from build123d import *

# Parameters (mm, degrees)
BOSS_EXTRUDE1_DEPTH     = 760
LPATTERN1_COUNT         = 2
LPATTERN1_PITCH         = 80
LPATTERN2_COUNT         = 9
LPATTERN2_PITCH         = 160
CUT_EXTRUDE1_DEPTH      = 40
CUT_EXTRUDE1_DEPTH_BACK = 20
SKETCH5_W               = 307.175258626
SKETCH5_H               = 1220.849909684


with BuildPart() as part:
    # Sketch1 → Boss-Extrude1 (new, symmetric)
    with BuildSketch(Plane.XY):
        with BuildLine():
            Line((-9.911771432, 13.106808119), (-11.43, 12.7))
            Line((-11.43, 12.7), (-14, 10.13))
            Line((-14, 10.13), (-14, 1.5))
            Line((-14, 1.5), (-12.5, 0))
            Line((-12.5, 0), (12.5, 0))
            Line((12.5, 0), (14, 1.5))
            Line((14, 1.5), (14, 10.13))
            Line((14, 10.13), (11.43, 12.7))
            Line((11.43, 12.7), (9.911771432, 13.106808119))
            ThreePointArc((9.911771432, 13.106808119), (9.10996999, 13.642554715), (8.8, 14.555696858))
            Line((8.8, 14.555696858), (8.8, 20.444303142))
            ThreePointArc((8.8, 20.444303142), (9.10996999, 21.357445285), (9.911771432, 21.893191881))
            Line((9.911771432, 21.893191881), (11.43, 22.3))
            Line((11.43, 22.3), (14, 24.87))
            Line((14, 24.87), (14, 26.5))
            ThreePointArc((14, 26.5), (13.416985894, 27.416985894), (12.5, 28))
            Line((12.5, 28), (-12.5, 28))
            ThreePointArc((-12.5, 28), (-13.416985894, 27.416985894), (-14, 26.5))
            Line((-14, 26.5), (-14, 24.87))
            Line((-14, 24.87), (-11.43, 22.3))
            Line((-11.43, 22.3), (-9.911771432, 21.893191881))
            ThreePointArc((-9.911771432, 21.893191881), (-9.10996999, 21.357445285), (-8.8, 20.444303142))
            Line((-8.8, 20.444303142), (-8.8, 14.555696858))
            ThreePointArc((-8.8, 14.555696858), (-9.10996999, 13.642554715), (-9.911771432, 13.106808119))
        make_face()
    extrude(amount=BOSS_EXTRUDE1_DEPTH, both=True)

    # Sketch2 → Cut-Revolve1 (revolve, cut)
    with BuildSketch(Plane(origin=(0, 0, 0), x_dir=(0, 0, -1), z_dir=(1, 0, 0)), mode=Mode.PRIVATE) as cut_revolve1_sk:
        Polygon((-720, 28), (-713, 28), (-713, 16), (-715.5, 16), (-715.5, 0), (-720, 0), align=None)
    cut_revolve1 = revolve(cut_revolve1_sk.sketch.rotate(Axis((0, 28, 720), (0, -1, 0)), 180), axis=Axis((0, 28, 720), (0, -1, 0)), mode=Mode.SUBTRACT)

    # LPattern1: Cut-Revolve1 ×2
    with Locations(*[(0, 0, -i * LPATTERN1_PITCH) for i in range(1, LPATTERN1_COUNT)]):
        add(cut_revolve1, mode=Mode.SUBTRACT)

    # Mirror1: Cut-Revolve1 across plane
    add(cut_revolve1.mirror(Plane.XY), mode=Mode.SUBTRACT)

    # Mirror1 copy 1 sketch → Mirror1 copy 1 (revolve, cut)
    with BuildSketch(Plane(origin=(0, 0, 80), x_dir=(0, 0, 1), z_dir=(1, 0, 0))):
        Polygon((-720, -28), (-713, -28), (-713, -16), (-715.5, -16), (-715.5, 0), (-720, 0), align=None)
    revolve(axis=Axis((0, 28, -640), (0, 1, 0)), mode=Mode.SUBTRACT)

    # LPattern2: Cut-Revolve1 ×9
    with Locations(*[(0, 0, -i * LPATTERN2_PITCH) for i in range(1, LPATTERN2_COUNT)]):
        add(cut_revolve1, mode=Mode.SUBTRACT)

    # LPattern2 copy 1 sketch → LPattern2 copy 1 (revolve, cut)
    with BuildSketch(Plane(origin=(0, 0, -240), x_dir=(0, 0, -1), z_dir=(1, 0, 0))):
        Polygon((-720, 28), (-713, 28), (-713, 16), (-715.5, 16), (-715.5, 0), (-720, 0), align=None)
    revolve(axis=Axis((0, 28, 480), (0, -1, 0)), mode=Mode.SUBTRACT)

    # LPattern2 copy 2 sketch → LPattern2 copy 2 (revolve, cut)
    with BuildSketch(Plane(origin=(0, 0, -400), x_dir=(0, 0, -1), z_dir=(1, 0, 0))):
        Polygon((-720, 28), (-713, 28), (-713, 16), (-715.5, 16), (-715.5, 0), (-720, 0), align=None)
    revolve(axis=Axis((0, 28, 320), (0, -1, 0)), mode=Mode.SUBTRACT)

    # LPattern2 copy 3 sketch → LPattern2 copy 3 (revolve, cut)
    with BuildSketch(Plane(origin=(0, 0, -560), x_dir=(0, 0, -1), z_dir=(1, 0, 0))):
        Polygon((-720, 28), (-713, 28), (-713, 16), (-715.5, 16), (-715.5, 0), (-720, 0), align=None)
    revolve(axis=Axis((0, 28, 160), (0, -1, 0)), mode=Mode.SUBTRACT)

    # LPattern2 copy 4 sketch → LPattern2 copy 4 (revolve, cut)
    with BuildSketch(Plane(origin=(0, 0, -720), x_dir=(0, 0, -1), z_dir=(1, 0, 0))):
        Polygon((-720, 28), (-713, 28), (-713, 16), (-715.5, 16), (-715.5, 0), (-720, 0), align=None)
    revolve(axis=Axis((0, 28, 0), (0, -1, 0)), mode=Mode.SUBTRACT)

    # LPattern2 copy 5 sketch → LPattern2 copy 5 (revolve, cut)
    with BuildSketch(Plane(origin=(0, 0, -880), x_dir=(0, 0, -1), z_dir=(1, 0, 0))):
        Polygon((-720, 28), (-713, 28), (-713, 16), (-715.5, 16), (-715.5, 0), (-720, 0), align=None)
    revolve(axis=Axis((0, 28, -160), (0, -1, 0)), mode=Mode.SUBTRACT)

    # LPattern2 copy 6 sketch → LPattern2 copy 6 (revolve, cut)
    with BuildSketch(Plane(origin=(0, 0, -1040), x_dir=(0, 0, -1), z_dir=(1, 0, 0))):
        Polygon((-720, 28), (-713, 28), (-713, 16), (-715.5, 16), (-715.5, 0), (-720, 0), align=None)
    revolve(axis=Axis((0, 28, -320), (0, -1, 0)), mode=Mode.SUBTRACT)

    # LPattern2 copy 7 sketch → LPattern2 copy 7 (revolve, cut)
    with BuildSketch(Plane(origin=(0, 0, -1200), x_dir=(0, 0, -1), z_dir=(1, 0, 0))):
        Polygon((-720, 28), (-713, 28), (-713, 16), (-715.5, 16), (-715.5, 0), (-720, 0), align=None)
    revolve(axis=Axis((0, 28, -480), (0, -1, 0)), mode=Mode.SUBTRACT)

    # LPattern2 copy 8 sketch → LPattern2 copy 8 (revolve, cut)
    with BuildSketch(Plane(origin=(0, 0, -1360), x_dir=(0, 0, -1), z_dir=(1, 0, 0))):
        Polygon((-720, 28), (-713, 28), (-713, 16), (-715.5, 16), (-715.5, 0), (-720, 0), align=None)
    revolve(axis=Axis((0, 28, -640), (0, -1, 0)), mode=Mode.SUBTRACT)

    # Sketch5 → Cut-Extrude1 (cut, two sides: drawn at the far end of the back side and taken through both)
    with BuildSketch(Plane(origin=(0, 0, 0), x_dir=(1, 0, 0), z_dir=(0, 1, 0)).offset(-CUT_EXTRUDE1_DEPTH_BACK)):
        with Locations((39.746319407, 155.224954842)):
            Rectangle(SKETCH5_W, SKETCH5_H)
    extrude(amount=CUT_EXTRUDE1_DEPTH + CUT_EXTRUDE1_DEPTH_BACK, mode=Mode.SUBTRACT)


solid = part.part
Build history of the part. All positions in model axes, mm. A direction names the side the tool comes from. Round coordinates to 2 decimals unless told otherwise and drop trailing zeros. Write each loop counter-clockwise with the first axis right and the second up, starting at its lowest first coordinate (ties: lowest second). Pieces come first, ordered by that corner, then holes. Notation, with made-up numbers: M 88.25,-26.75 L 143.25,-26.75 A22 cw 143.25,10.25 Z; hole C -11,-21.75 d9. An arc over 180 degrees is marked long. Answer as a JSON object with one key per item and string values. Group by question number.
(1) Cut at B-B (y = 6). Give the cut face in (x, z).
(2) Mould opens along Z. For faces 4 (the flat face through (0, 14, 760)), 5 (the flat face through (-8.8, 18, 610)), 6 (the flat face through (5, 16, 720)) say: pulls with the +Z half, pulls with the -Z half, needs draft (parallel to the pull), parting line crosses it, or undercut.
(3) Cut at D-D (z = 730). Give the cut face in (x, y), and give its area (3 significant figures).
(4) Which spindle directions (+Z, -Z, +X, -X, +Y, -Y) get a long thin tool onto all of the face, cutting with end or side? Do faces 1 (the flat face through (0, 14, 455.2)), 2 (the flat face through (8.8, 17, 610)), 3 (the flat face through (5, 16, 640)). Say none if no direction does.
(5) Cut at C-C (x = 0). Give the number of separate pieces and of enclosed holes in the cut face, and give its area (3 significant figures).
(6) Drill centre lines: L1, parallel to Y at x = 11.25, z = 711; L2, parallel to X at y = 19.75, z = 720; L3, parallel to X at y = 10, z = 480. Where is each one in solid material? Low to high.
(7) Flat gauge pins, fed straight in: pin 1 (12.5 mm diameter, centred on x = 0, z = 560, fed in from +Y); pin 2 (7 mm diameter, centred on x = 0, z = 560, fed in from -Y) (3 decimals); pin 3 (1.8 mm diameter, centred on y = 17, z = 542.5, fed in from +X); pin 4 (16 mm diameter, centred on x = 0, z = 640, fed in from +Y). Where does each tip first touch, or does it go through?
Responses:
{
 "1": {"outline": "M -14,455.2 L 14,455.2 L 14,760 L -14,760 Z; hole C 0,480 d9; hole C 0,560 d9; hole C 0,640 d9; hole C 0,720 d9"},
 "2": {"face 4": "pulls with the +Z half", "face 5": "needs draft", "face 6": "undercut"},
 "3": {"outline": "M -14,1.5 L -12.5,0 L 12.5,0 L 14,1.5 L 14,10.13 L 11.43,12.7 L 9.91,13.11 A1.5 cw 8.8,14.56 L 8.8,20.44 A1.5 cw 9.91,21.89 L 11.43,22.3 L 14,24.87 L 14,26.5 A2.5 ccw 12.5,28 L -12.5,28 A2.5 ccw -14,26.5 L -14,24.87 L -11.43,22.3 L -9.91,21.89 A1.5 cw -8.8,20.44 L -8.8,14.56 A1.5 cw -9.91,13.11 L -11.43,12.7 L -14,10.13 Z", "area": "672 mm2"},
 "4": {"face 1": "-Z, +X, -X, +Y, -Y", "face 2": "+Z, -Z, +X", "face 3": "+Y"},
 "5": {"separate pieces": "5", "enclosed holes": "0", "area": "7,290 mm2"},
 "6": {"L1": "y = 0 to 12.75, 22.25 to 28", "L2": "x = -8.8 to -7, 7 to 8.8", "L3": "x = -14 to -4.5, 4.5 to 14"},
 "7": {"pin 1": "stops at y = 16", "pin 2": "passes through", "pin 3": "stops at x = 8.8", "pin 4": "stops at y = 28"}
}
